from build123d import *

# Parameters (mm, degrees)
F0_W     = 120.1
F0_H     = 71.1
F0_R     = 5
F0_R_2   = 3
F0_W_2   = 64.3
F0_H_2   = 15.9
F1_DEPTH = 1


with BuildPart() as f1:
    # F0 (on Top) → F1 (new body)
    with BuildSketch(Plane.XY):
        with Locations((60.05, 35.55)):
            Rectangle(F0_W, F0_H)
        with Locations((35, 13.2)):
            Circle(F0_R, mode=Mode.SUBTRACT)
        with Locations((70.2, 13.2)):
            Circle(F0_R_2, mode=Mode.SUBTRACT)
        with Locations((95.8, 13.2)):
            Circle(F0_R_2, mode=Mode.SUBTRACT)
        with Locations((111.1, 34.4)):
            Circle(F0_R_2, mode=Mode.SUBTRACT)
        with Locations((59.35, 45.85)):
            Rectangle(F0_W_2, F0_H_2, mode=Mode.SUBTRACT)
        with Locations((10, 56.6)):
            Circle(F0_R_2, mode=Mode.SUBTRACT)
        with Locations((111.1, 56.6)):
            Circle(F0_R_2, mode=Mode.SUBTRACT)
    extrude(amount=F1_DEPTH)


solid = f1.part
Work out the finished part from the listing and answer in its coordinate system (mm). Round coordinates to 2 decimals unless told otherwise and drop trailing zeros. Write each loop counter-clockwise with the first axis right and the second up, starting at its lowest first coordinate (ties: lowest second). Pieces come first, ordered by that corner, then holes.
1) A cutting plane is placed at B-B (y = 50). Give the vertices of the cut face in (x, z).
2) A cutting plane is placed at D-D (x = 111.1). Give the vertices of the cut face in (y, z), plus the area to 3 significant figures.
3) A cutting plane is placed at A-A (x = 59). Give the vertices of the cut face in (y, z), plus the area to 3 significant figures.
4) A cutting plane is placed at C-C (z = 0.7). Give the vertices of the cut face in (x, y).
5) Straight lines are drawn through the part: line 1 (Y direction, x = 111.1, z = 0.55); line 2 (Y direction, x = 53.5, z = 0.2); line 3 (X direction, y = 42.5, z = 0.45). For each, find the intervals that lie inside material, in ascending order.
6) The mould has two halves that part along X. Classify faces 1 (the flat face through (59, 36, 0)), 2 (the cylindrical face through (30.005, 13.42, 0.493)): pulls with the +X half, pulls with the -X half, needs draft (parallel to the pull), parting line crosses it, or undercut.
Completed:
1. outline: (0, 0) - (27.2, 0) - (27.2, 1) - (0, 1) - close; (91.5, 0) - (120.1, 0) - (120.1, 1) - (91.5, 1) - close
2. outline: (0, 0) - (31.4, 0) - (31.4, 1) - (0, 1) - close; (37.4, 0) - (53.6, 0) - (53.6, 1) - (37.4, 1) - close; (59.6, 0) - (71.1, 0) - (71.1, 1) - (59.6, 1) - close
2. area: 59.1 mm2
3. outline: (0, 0) - (37.9, 0) - (37.9, 1) - (0, 1) - close; (53.8, 0) - (71.1, 0) - (71.1, 1) - (53.8, 1) - close
3. area: 55.2 mm2
4. outline: (0, 0) - (120.1, 0) - (120.1, 71.1) - (0, 71.1) - close; hole circle Ø6 at (10, 56.6); hole (27.2, 37.9) - (91.5, 37.9) - (91.5, 53.8) - (27.2, 53.8) - close; hole circle Ø10 at (35, 13.2); hole circle Ø6 at (70.2, 13.2); hole circle Ø6 at (95.8, 13.2); hole circle Ø6 at (111.1, 34.4); hole circle Ø6 at (111.1, 56.6)
5. line 1: y = 0 to 31.4, 37.4 to 53.6, 59.6 to 71.1
5. line 2: y = 0 to 37.9, 53.8 to 71.1
5. line 3: x = 0 to 27.2, 91.5 to 120.1
6. face 1: needs draft
6. face 2: undercut
